```python
from build123d import *

# Parameters (mm, degrees)
F1_DEPTH = 3
F3_DEPTH = 3.001
F4_R     = 5
F5_DEPTH = 3.001
F7_DEPTH = 3.001
F9_DEPTH = 3.001


with BuildPart() as f1:
    # F0 (on Top) → F1 (new body)
    with BuildSketch(Plane.XY):
        with BuildLine():
            Line((0, 0), (51.4312095756, 70.7889870078))
            ThreePointArc((51.4312095756, 70.7889870078), (0, 87.5), (-51.4312095756, 70.7889870078))
            Line((-51.4312095756, 70.7889870078), (0, 0))
        make_face()
    extrude(amount=F1_DEPTH)

    # F2 (on face) → F3 (cut, through all)
    with BuildSketch(Plane.XY.offset(3)):
        with BuildLine():
            Line((0, 0), (23.5114100917, 32.360679775))
            ThreePointArc((23.5114100917, 32.360679775), (0, 40), (-23.5114100917, 32.360679775))
            Line((-23.5114100917, 32.360679775), (0, 0))
        make_face()
    extrude(amount=-F3_DEPTH, mode=Mode.SUBTRACT)

    # F4 (on face) → F5 (cut, through all)
    with BuildSketch(Plane.XY.offset(3)):
        with Locations((0, 48)):
            Circle(F4_R)
    extrude(amount=-F5_DEPTH, mode=Mode.SUBTRACT)

    # F6 (on face) → F7 (cut, through all)
    with BuildSketch(Plane.XY.offset(3)):
        with BuildLine():
            ThreePointArc((-23.5114100917, 32.360679775), (-16.5886439103, 36.3980341944), (-9, 38.9743505398))
            Line((-9, 38.9743505398), (-28.3165231686, 38.9743505398))
            Line((-28.3165231686, 38.9743505398), (-23.5114100917, 32.360679775))
        make_face()
        with BuildLine():
            Line((28.3165231686, 38.9743505398), (9, 38.9743505398))
            ThreePointArc((9, 38.9743505398), (16.5886439103, 36.3980341944), (23.5114100917, 32.360679775))
            Line((23.5114100917, 32.360679775), (28.3165231686, 38.9743505398))
        make_face()
    extrude(amount=-F7_DEPTH, mode=Mode.SUBTRACT)

    # F8 (on face) → F9 (cut, through all)
    with BuildSketch(Plane.XY.offset(3)):
        Polygon((-28.3165231686, 38.9743505398), (-9, 38.9743505398), (-9, 42.9743505398), (-31.2226932806, 42.9743505398), align=None)
        Polygon((9, 42.9743505398), (9, 38.9743505398), (28.3165231686, 38.9743505398), (31.2226932806, 42.9743505398), align=None)
    extrude(amount=-F9_DEPTH, mode=Mode.SUBTRACT)


solid = f1.part
```
Design review of the part built by this model. Coordinates are the model's own, in mm. A direction names the side the tool comes from. Round coordinates to 2 decimals unless told otherwise and drop trailing zeros. Write each loop counter-clockwise with the first axis right and the second up, starting at its lowest first coordinate (ties: lowest second). Pieces come first, ordered by that corner, then holes. Notation, with made-up numbers: (16, 76.5) -> (29, 76.5) arc R14 cw to (29, 85.5) -> close; hole circle Ø8 at (7, -24.5). An arc over 180 degrees is marked (long way). Answer in a Markdown table with one row per item.
Q1. To check wall thickness, follow L1, parallel to Y at x = 0, z = 1.2; L2, parallel to X at y = 44, z = 0.9; L3, parallel to Y at x = 14, z = 0.9. State the ranges of each line that lie inside material, in increasing order. Write a range as [from, to].
The answers:
| item | result |
|---|---|
| L1 | [40, 43], [53, 87.5] |
| L2 | [-31.97, -3], [3, 31.97] |
| L3 | [42.97, 86.37] |
Q2. Take a section at C-C, the plane z = 0.9. State the section outline as (x, y) points.
The answers:
| item | result |
|---|---|
| outline | (-51.43, 70.79) -> (-31.22, 42.97) -> (-9, 42.97) -> (-9, 38.97) arc R40 cw to (9, 38.97) -> (9, 42.97) -> (31.22, 42.97) -> (51.43, 70.79) arc R87.5 ccw to start; hole circle Ø10 at (0, 48) |
Q3. Take a section at D-D, the plane y = 61. State the section outline as (x, z) points.
The answers:
| item | result |
|---|---|
| outline | (-44.32, 0) -> (44.32, 0) -> (44.32, 3) -> (-44.32, 3) -> close |
Q4. Take a section at A-A, the plane x = 0. State the section outline as (y, z) points, then the cut area to 4 significant figures.
The answers:
| item | result |
|---|---|
| outline | (40, 0) -> (43, 0) -> (43, 3) -> (40, 3) -> close; (53, 0) -> (87.5, 0) -> (87.5, 3) -> (53, 3) -> close |
| area | 112.5 mm² |
Q5. For faces 4 (the face through (-20, 42.974, 2)), 5 (the face through (-1, 64, 3)), 6 (the face through (20, 42.974, 2)), list the 3-axis set-ups (+Z, -Z, +X, -X, +Y, -Y) from which the entire face can be reached by the end or side of a thin tool; tool diameter is ignored.
The answers:
| item | result |
|---|---|
| face 4 | +Z, -Z, -X, -Y |
| face 5 | +Z, +X, -X, +Y, -Y |
| face 6 | +Z, -Z, +X, -Y |
Q6. Take a section at B-B, the plane y = 46. State the section outline as (x, z) points.
The answers:
| item | result |
|---|---|
| outline | (-33.42, 0) -> (-4.58, 0) -> (-4.58, 3) -> (-33.42, 3) -> close; (4.58, 0) -> (33.42, 0) -> (33.42, 3) -> (4.58, 3) -> close |
Q7. Clearance check with flat-ended pins moving along their axes: pin 1 Ø1.5 at (y, z) = (41, 1.5) entering from -X; pin 2 Ø1.5 at (x, z) = (16, 1.5) entering from -Y. State where each tip first meets the part, or that it passes through.
The answers:
| item | result |
|---|---|
| pin 1 | x = -9 |
| pin 2 | y = 42.97 |
Q8. Draft analysis for pull direction X (two halves, no side actions). For faces 1 (the face through (-1, 64, 0)), 2 (the face through (-0.651, 52.957, 1.521)), 3 (the face through (0.77, 87.497, 1.479)), state which applies: +X half, -X half, draft (parallel to the pull), parting line (faces both ways), or undercut.
The answers:
| item | result |
|---|---|
| face 1 | draft |
| face 2 | undercut |
| face 3 | parting line |
